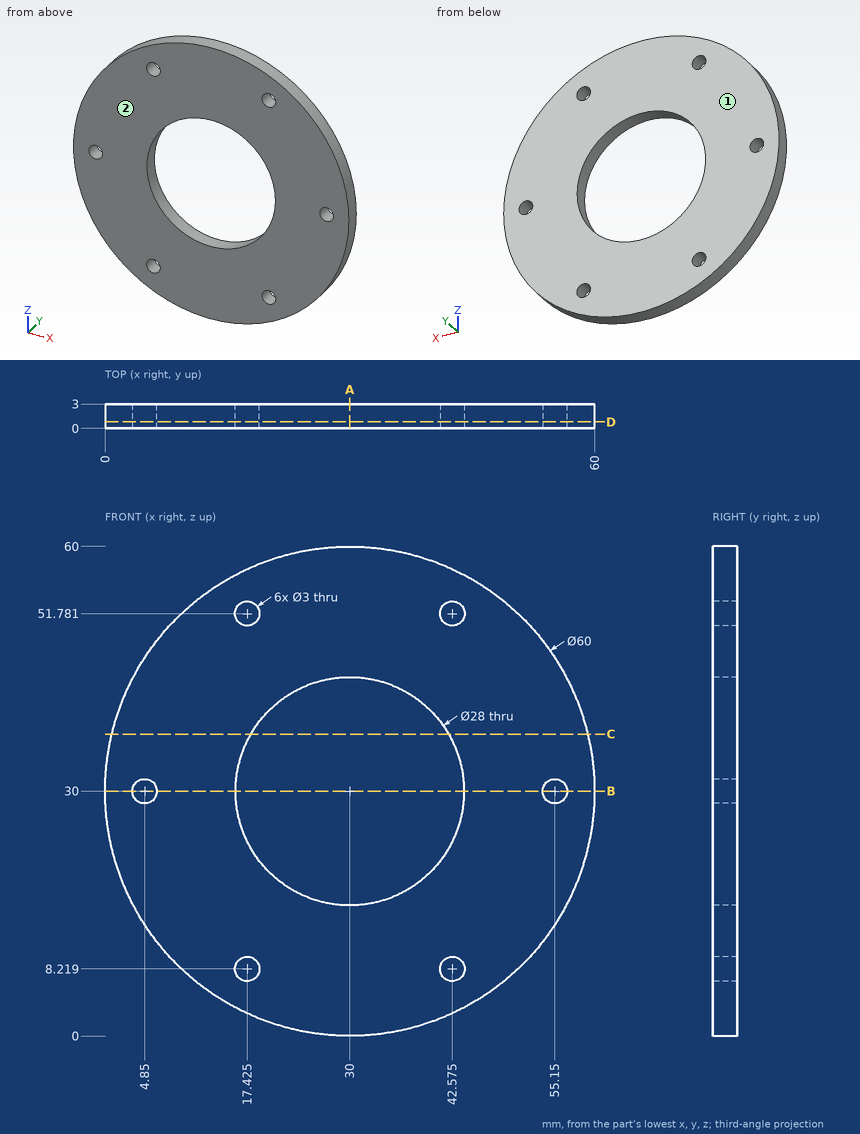
Could you check a few things on this drawing? It's one solid part, dimensions in mm from its lowest x, y, z. Give positions to 0.01 mm unless a question says otherwise; leave off trailing zeros. Order: outer loops, then holes, each group sorted by start corner. A loop starts at its lowest first (then second) coordinate and runs counter-clockwise, first axis right, second up. Notation, with made-up numbers: (58.25, 9) - (97.25, 9) arc R28 cw to (97.25, 36) - close; hole circle Ø2 at (63.5, 63). An arc over 180 degrees is marked (long way). Answer as a JSON object with one key per item and string values. Group by question number.
Item 1: If we section it at B-B on z = 30: Please give me the cut outline in (x, y).
Item 2: If we section it at C-C on z = 37: Please give me the cut outline in (x, y) (1 decimal), and give its area (3 significant figures).
Item 3: Please list where these lines run through material, in increasing order: probe 1 along Z at (x, y) = (42.5, 0.5) (1 decimal); probe 2 along X at (y, z) = (1.9, 52) (1 decimal); probe 3 along Z at (x, y) = (30, 1.5).
Item 4: If we section it at D-D on y = 0.8: Give the number of separate pieces and of enclosed holes in the cut face, and give its area (3 significant figures).
Item 5: If we section it at A-A on x = 30: Please give me the cut outline in (y, z).
Item 6: For P1, Ø1, axis at x = 37.5, y = 0.5, coming from the +Z side, with a flat end and sliding along its axis, tell me the tip position at first contact or that it passes through.
Item 7: If we mould it in two halves opening along Y, with no side actions, what happens to the marked faces 1 and 2? For each: pulls with the +Y half, pulls with the -Y half, needs draft (parallel to the pull), parting line crosses it, or undercut.
Result set:
{
 "1": {"outline": "(0, 0) - (3.35, 0) - (3.35, 3) - (0, 3) - close; (6.35, 0) - (16, 0) - (16, 3) - (6.35, 3) - close; (44, 0) - (53.65, 0) - (53.65, 3) - (44, 3) - close; (56.65, 0) - (60, 0) - (60, 3) - (56.65, 3) - close"},
 "2": {"outline": "(0.8, 0) - (17.9, 0) - (17.9, 3) - (0.8, 3) - close; (42.1, 0) - (59.2, 0) - (59.2, 3) - (42.1, 3) - close", "area": "102 mm²"},
 "3": {"probe 1": "2.7 to 6.7, 9.7 to 23.7, 36.3 to 50.3, 53.3 to 57.3", "probe 2": "9.6 to 15.9, 18.9 to 41.1, 44.1 to 50.4", "probe 3": "0 to 16, 44 to 60"},
 "4": {"separate pieces": "1", "enclosed holes": "7", "area": "2,170 mm²"},
 "5": {"outline": "(0, 0) - (3, 0) - (3, 16) - (0, 16) - close; (0, 44) - (3, 44) - (3, 60) - (0, 60) - close"},
 "6": {"P1": "z = 59.17"},
 "7": {"face 1": "pulls with the +Y half", "face 2": "pulls with the -Y half"}
}
